from build123d import *

# Parameters (mm, degrees)
BOX_W           = 32
BOX_H           = 9.8
BOX_DEPTH       = 9.8
CHAMFER_SIZE    = 2
CHAMFER001_SIZE = 1
CHAMFER002_SIZE = 1


with BuildPart() as part:
    # Box → Box (new body)
    with BuildSketch(Plane.XY):
        with Locations((16, 4.9)):
            Rectangle(BOX_W, BOX_H)
    extrude(amount=BOX_DEPTH)

    # Chamfer
    chamfer_edges = [part.edges().sort_by_distance(p)[0] for p in [
        (16, 0, 0),
        (16, 0, 9.8),
        (16, 9.8, 0),
        (16, 9.8, 9.8),
    ]]
    chamfer(chamfer_edges, length=CHAMFER_SIZE)

    # Chamfer001
    chamfer001_edges = [part.edges().sort_by_distance(p)[0] for p in [
        (0, 0, 4.9),
        (0, 1, 1),
        (0, 1, 8.8),
        (0, 4.9, 0),
        (0, 4.9, 9.8),
        (0, 8.8, 1),
        (0, 8.8, 8.8),
        (0, 9.8, 4.9),
    ]]
    chamfer(chamfer001_edges, length=CHAMFER001_SIZE)

    # Chamfer002
    chamfer002_edges = [part.edges().sort_by_distance(p)[0] for p in [
        (32, 0, 4.9),
        (32, 1, 1),
        (32, 1, 8.8),
        (32, 4.9, 0),
        (32, 4.9, 9.8),
        (32, 8.8, 1),
        (32, 8.8, 8.8),
        (32, 9.8, 4.9),
    ]]
    chamfer(chamfer002_edges, length=CHAMFER002_SIZE)


solid = part.part
Model file for the job. Use its own axes, mm. Round coordinates to 2 decimals unless told otherwise and drop trailing zeros. Order: outer loops, then holes, each group sorted by start corner. A loop starts at its lowest first (then second) coordinate and runs counter-clockwise, first axis right, second up.
(1) Pin check, flat tips, straight feed: pin 1 (1 mm diameter, centred on x = 12, y = 1, fed in from -Z); pin 2 (5 mm diameter, centred on x = 19, z = 8, fed in from -Y); pin 3 (1 mm diameter, centred on x = 26, y = 8.5, fed in from -Z). Stop position of each tip, or through.
(2) Band-saw the part on B-B (y = 9.25). List the corners of the cut face in (x, z).
(3) Drill centre lines: line 1 (Y direction, x = 17.5, z = 1); line 2 (Y direction, x = 14, z = 0.5); line 3 (Z direction, x = 13.5, y = 1.75). Where is each one in solid material? Low to high.
(4) Band-saw the part on A-A (x = 15.5). List the corners of the cut face in (y, z).
Verdict:
1. pin 1: stops at z = 0.5
1. pin 2: stops at y = 0
1. pin 3: stops at z = 0.2
2. outline: (0.45, 2.23) - (1, 1.45) - (31, 1.45) - (31.55, 2.23) - (31.55, 7.57) - (31, 8.35) - (1, 8.35) - (0.45, 7.57) - close
3. line 1: y = 1 to 8.8
3. line 2: y = 1.5 to 8.3
3. line 3: z = 0.25 to 9.55
4. outline: (0, 2) - (2, 0) - (7.8, 0) - (9.8, 2) - (9.8, 7.8) - (7.8, 9.8) - (2, 9.8) - (0, 7.8) - close
